Here's the drawing with two shaded views (mm, measured from the low corner). I have some questions. A direction names the side the tool comes from. Coordinates: 2 decimals unless noted, no trailing zeros. Order: outer loops, then holes, each group sorted by start corner. A loop starts at its lowest first (then second) coordinate and runs counter-clockwise, first axis right, second up. Notation, with made-up numbers: (7, 50.25) - (18, 50.25) arc R15 ccw to (18, 54.25) - close; hole circle Ø2 at (79.5, -33.5). An arc over 180 degrees is marked (long way). Answer as a JSON object with one key per item and string values. Group by question number.
(1) Please list where these lines run through material, in increasing order: probe 1 along Z at (x, y) = (143, 533.4); probe 2 along Y at (x, z) = (23.5, 34); probe 3 along X at (y, z) = (88, 46).
(2) Imagine slicing it at B-B, the plane y = 610. Write out the boundary of the cut face in (x, z), and give its area (3 significant figures).
(3) Imagine slicing it at A-A, the plane x = 119.5. Write out the boundary of the cut face in (y, z).
(4) Imagine slicing it at C-C, the plane z = 395.5. Write out the boundary of the cut face in (x, y), and give its area (3 significant figures).
(5) Imagine slicing it at D-D, the plane y = 201. Write out the boundary of the cut face in (x, z), and give its area (3 significant figures).
(6) Will this pin go through, and if not, where does the flat tip stop? P1, Ø1.5, axis at y = 851, z = 137, coming from the -X side.
(7) Which directions (+Z, -Z, +X, -X, +Y, -Y) give clear straight access to the entire face, cutting with the end or side of a thin tool? Please do the marked faces 5 and 6.
(8) We'd pull the mould along Y, two halves only. Please class the marked faces 1, 2, 3 and 4: pulls with the +Y half, pulls with the -Y half, needs draft (parallel to the pull), parting line crosses it, or undercut.
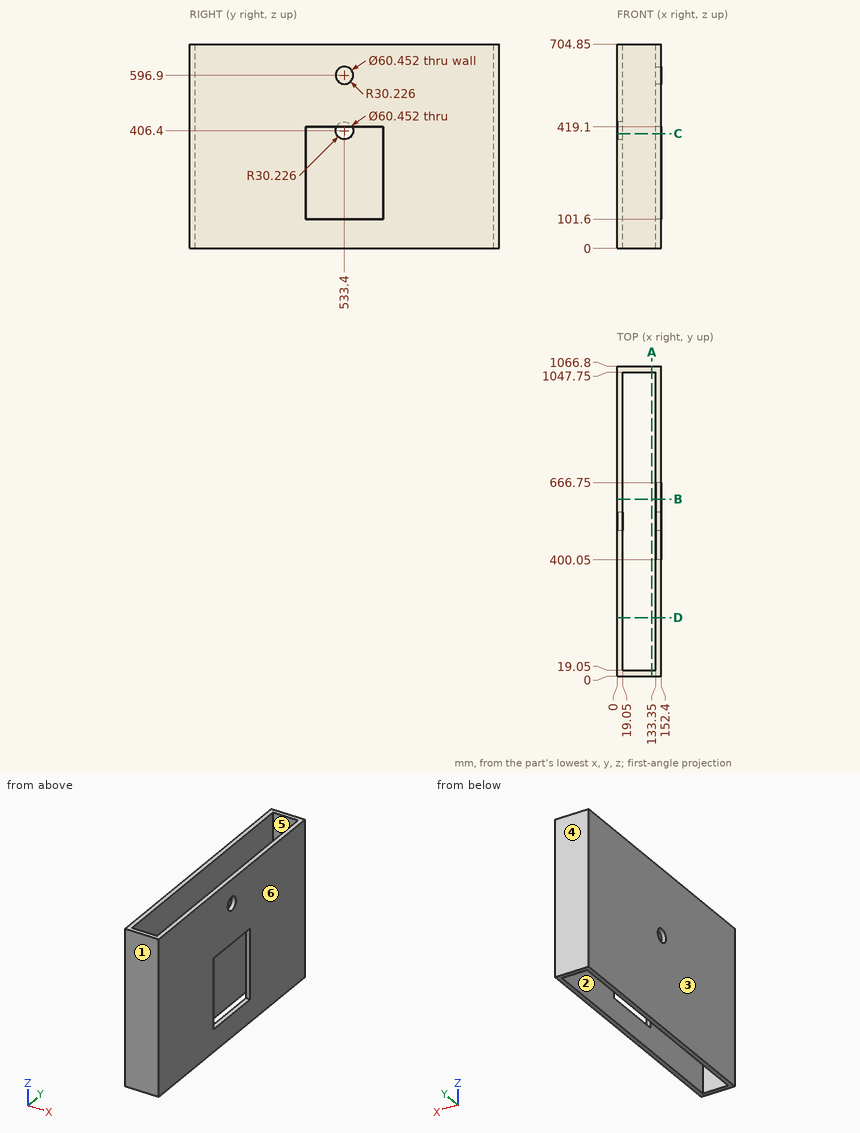
Result set:
{
 "1": {"probe 1": "z = 0 to 101.6, 419.1 to 566.67, 627.13 to 704.85", "probe 2": "y = 0 to 19.05, 1047.75 to 1066.8", "probe 3": "x = 0 to 19.05, 133.35 to 152.4"},
 "2": {"outline": "(0, 0) - (19.05, 0) - (19.05, 704.85) - (0, 704.85) - close; (133.35, 0) - (152.4, 0) - (152.4, 101.6) - (133.35, 101.6) - close; (133.35, 419.1) - (152.4, 419.1) - (152.4, 704.85) - (133.35, 704.85) - close", "area": "20,800 mm^2"},
 "3": {"outline": "(0, 0) - (19.05, 0) - (19.05, 704.85) - (0, 704.85) - close; (1047.75, 0) - (1066.8, 0) - (1066.8, 704.85) - (1047.75, 704.85) - close"},
 "4": {"outline": "(0, 0) - (152.4, 0) - (152.4, 400.05) - (133.35, 400.05) - (133.35, 19.05) - (19.05, 19.05) - (19.05, 505.21) - (0, 505.21) - close; (0, 561.59) - (19.05, 561.59) - (19.05, 1047.75) - (133.35, 1047.75) - (133.35, 666.75) - (152.4, 666.75) - (152.4, 1066.8) - (0, 1066.8) - close", "area": "38,800 mm^2"},
 "5": {"outline": "(0, 0) - (19.05, 0) - (19.05, 704.85) - (0, 704.85) - close; (133.35, 0) - (152.4, 0) - (152.4, 704.85) - (133.35, 704.85) - close", "area": "26,900 mm^2"},
 "6": {"P1": "stops at x = 0"},
 "7": {"face 5": "+Z, -Z", "face 6": "+Z, -Z, +X, +Y, -Y"},
 "8": {"face 1": "pulls with the -Y half", "face 2": "undercut", "face 3": "needs draft", "face 4": "pulls with the +Y half"}
}
